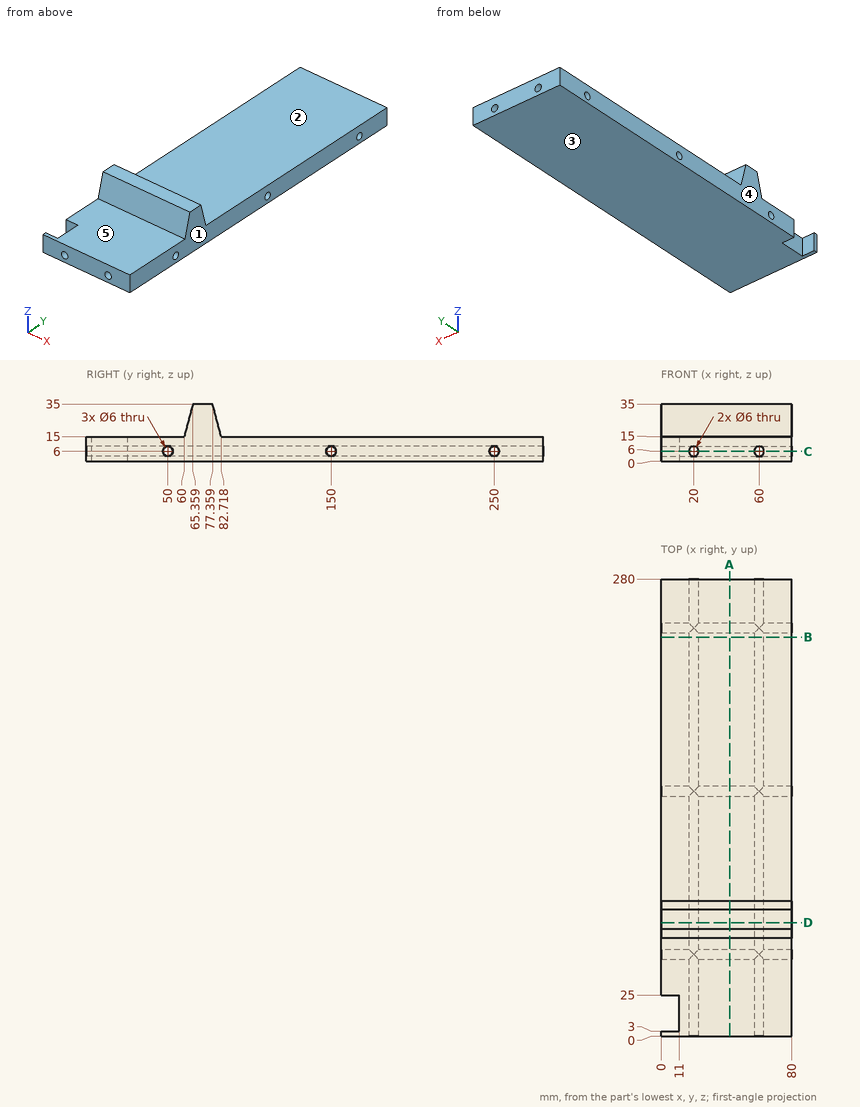
Source: three-view drawing plus pictorial views. Frame: mm from the lowest corner of the part. A direction names the side the tool comes from. Round coordinates to 2 decimals unless told otherwise and drop trailing zeros. Order: outer loops, then holes, each group sorted by start corner. A loop starts at its lowest first (then second) coordinate and runs counter-clockwise, first axis right, second up. Notation, with made-up numbers: (59, 23) - (101, 23) arc R7 cw to (101, 28) - close; hole circle Ø4 at (67, 54). An arc over 180 degrees is marked (long way). Write each question's results on one line, items separated by ' | '.
Item 1: Section C-C, the plane z = 6. State how many separate pieces and enclosed holes the cut face has, and give its area (3 significant figures).
Completed:
separate pieces: 12 | enclosed holes: 0 | area: 17,600 mm^2
Item 2: Mould query, pull axis Z, two halves, no side actions, for the marked faces 1, 2 and 3. Classes: pulls with the +Z half, pulls with the -Z half, needs draft (parallel to the pull), parting line crosses it, or undercut.
Completed:
face 1: needs draft | face 2: pulls with the +Z half | face 3: pulls with the -Z half
Item 3: Section D-D, the plane y = 69.5. Return the cut outline in (x, z), and give its area (3 significant figures).
Completed:
outline: (0, 0) - (80, 0) - (80, 35) - (0, 35) - close; hole circle Ø6 at (20, 6); hole circle Ø6 at (60, 6) | area: 2,740 mm^2
Item 4: Section B-B, the plane y = 244.5. Return the cut outline in (x, z), and give its area (3 significant figures).
Completed:
outline: (0, 0) - (80, 0) - (80, 15) - (0, 15) - close; hole circle Ø6 at (20, 6); hole circle Ø6 at (60, 6) | area: 1,140 mm^2
Item 5: Reachability of the marked faces 4 and 5 from +Z, -Z, +X, -X, +Y, -Y: full face, straight path, thin tool, end or side. Return the list, or none.
Completed:
face 4: +Z, -Z, -X, +Y, -Y | face 5: +Z, +X, -X, -Y
Item 6: Material intervals for line 1 along Y through (x, z) = (7.5, 6.5); line 2 along X through (y, z) = (119, 6); line 3 along Y through (x, z) = (66.25, 6), sorted ascending. Write a range as [from, to].
Completed:
line 1: [0, 3], [25, 47.04], [52.96, 147.04], [152.96, 247.04], [252.96, 280] | line 2: [0, 17], [23, 57], [63, 80] | line 3: [0, 47], [53, 147], [153, 247], [253, 280]
Item 7: First-contact query: pin 1 Ø1.5 at (x, y) = (11, 152) entering from +Z; pin 2 Ø7 at (y, z) = (50, 6) entering from +X; pin 3 Ø3 at (x, z) = (16.5, 20) entering from +Y; pin 4 Ø7.5 at (y, z) = (9, 6.5) entering from -X. Flat tips, straight axial feed; report the tip coordinate or a pass-through.
Completed:
pin 1: z = 15 | pin 2: x = 80 | pin 3: y = 81.78 | pin 4: x = 11
Item 8: Section A-A, the plane x = 42. Return the cut outline in (y, z).
Completed:
outline: (0, 0) - (280, 0) - (280, 15) - (82.72, 15) - (77.36, 35) - (65.36, 35) - (60, 15) - (0, 15) - close; hole circle Ø6 at (50, 6); hole circle Ø6 at (150, 6); hole circle Ø6 at (250, 6)
